Job drawing, mm, ordinate dimensions from the low corner. One solid piece. A direction names the side the tool comes from. Give positions to 0.01 mm unless a question says otherwise; leave off trailing zeros. Loops run counter-clockwise (first coordinate to the right, second up) from the corner with the lowest first, then second, coordinate; pieces in that order, holes last. Notation, with made-up numbers: M 29,22.25 L 53,22.25 A9 cw 53,33.25 Z; hole C 76.5,42.25 d1. An arc over 180 degrees is marked long. Put each result on its own line as item: value.
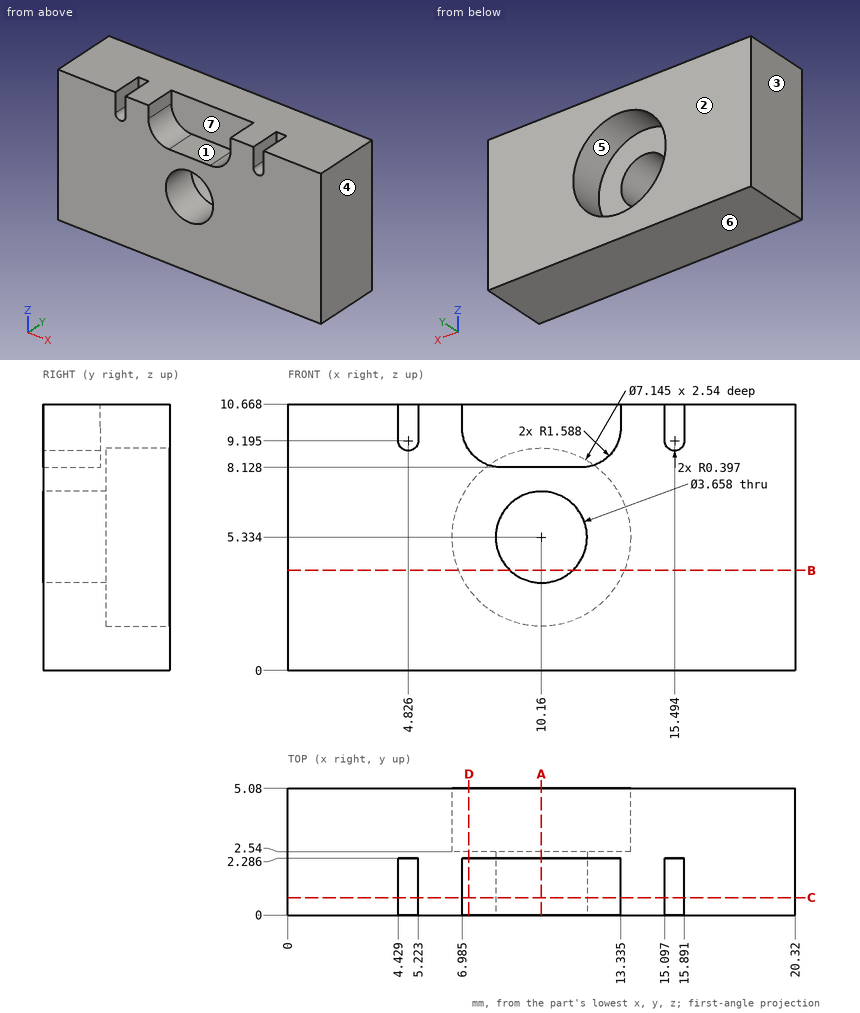
Q1. Slice it at D-D (x = 7.25). List the corners of the cut face in (y, z) (1 decimal).
Here are the results:
outline: M 0,0 L 5.1,0 L 5.1,3.3 L 2.5,3.3 L 2.5,7.4 L 5.1,7.4 L 5.1,10.7 L 2.3,10.7 L 2.3,8.8 L 0,8.8 Z
Q2. Tool access for the marked faces 5, 6 and 7: list every direction of +Z, -Z, +X, -X, +Y, -Y with a clear straight run to the whole face (end or side of a thin tool).
Here are the results:
face 5: +Y
face 6: -Z, +X, -X, +Y, -Y
face 7: +Z, -Y
Q3. Slice it at B-B (z = 4). List the corners of the cut face in (x, y) (1 decimal).
Here are the results:
outline: M 0,0 L 8.9,0 L 8.9,2.5 L 6.8,2.5 L 6.8,5.1 L 0,5.1 Z; M 11.4,0 L 20.3,0 L 20.3,5.1 L 13.5,5.1 L 13.5,2.5 L 11.4,2.5 Z
Q4. Mould opens along X. For the marked faces 1, 2, 3 and 4 say: pulls with the +X half, pulls with the -X half, needs draft (parallel to the pull), parting line crosses it, or undercut.
Here are the results:
face 1: undercut
face 2: needs draft
face 3: pulls with the -X half
face 4: pulls with the +X half
Q5. Drop flat-ended pins along their axis: pin 1 Ø2 at (x, z) = (10.16, 5.334) entering from -Y; pin 2 Ø1.5 at (x, y) = (8.5, 1.5) entering from +Z; pin 3 Ø5.5 at (x, z) = (10.16, 5.334) entering from +Y. Give the stop position or say it passes through.
Here are the results:
pin 1: through
pin 2: z = 8.36
pin 3: y = 2.54
Q6. Slice it at A-A (x = 10.16). List the corners of the cut face in (y, z) (1 decimal).
Here are the results:
outline: M 0,0 L 5.1,0 L 5.1,1.8 L 2.5,1.8 L 2.5,3.5 L 0,3.5 Z; M 0,7.2 L 2.5,7.2 L 2.5,8.9 L 5.1,8.9 L 5.1,10.7 L 2.3,10.7 L 2.3,8.1 L 0,8.1 Z
Q7. Slice it at C-C (y = 0.7). List the corners of the cut face in (x, z) (1 decimal), and give its area (3 significant figures).
Here are the results:
outline: M 0,0 L 20.3,0 L 20.3,10.7 L 15.9,10.7 L 15.9,9.2 A0.4 cw 15.1,9.2 L 15.1,10.7 L 13.3,10.7 L 13.3,9.7 A1.6 cw 11.7,8.1 L 8.6,8.1 A1.6 cw 7,9.7 L 7,10.7 L 5.2,10.7 L 5.2,9.2 A0.4 cw 4.4,9.2 L 4.4,10.7 L 0,10.7 Z; hole C 10.2,5.3 d3.7
area: 188 mm²
Q8. Probe line 1 (Z direction, x = 10.16, y = 0.6) (1 decimal); line 2 (X direction, y = 1.7, z = 9.5); line 3 (Y direction, x = 12.5, z = 5.5). List the from-to ranges inside material, lowest first. Write a range as from..to.
Here are the results:
line 1: 0..3.5, 7.2..8.1
line 2: 0..4.43, 5.22..7, 13.32..15.1, 15.89..20.32
line 3: 0..2.54
